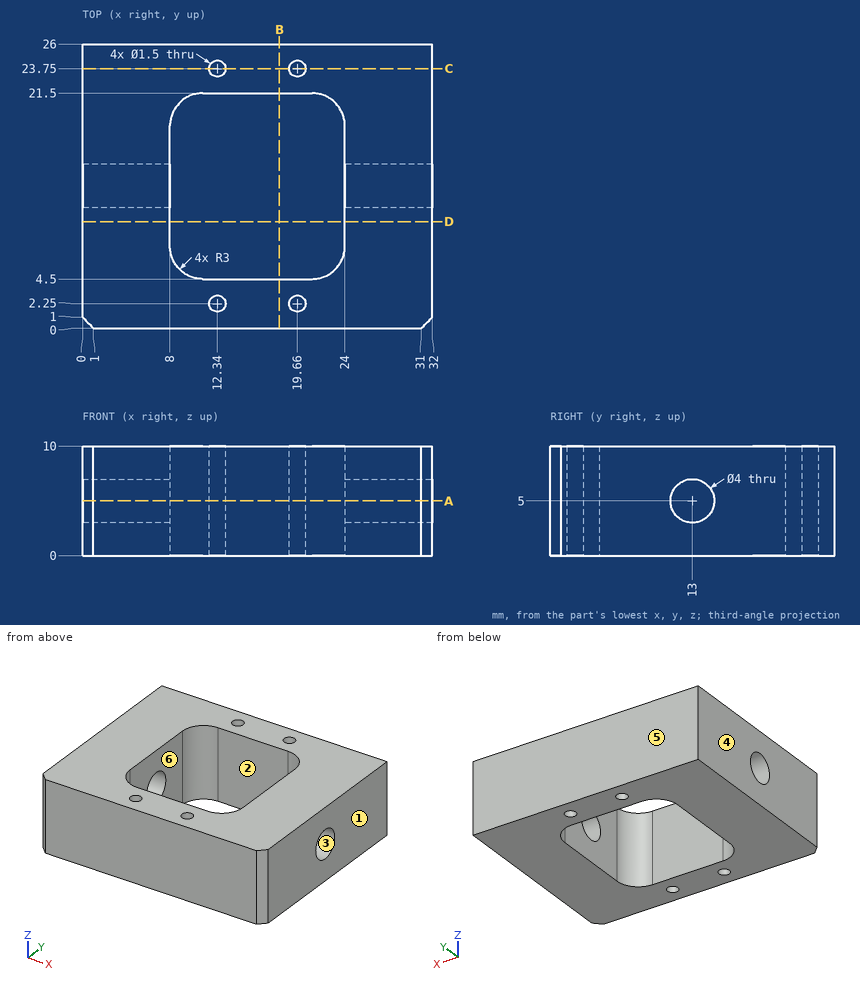
Can you work these out from the drawing? Everything is in mm from the part's minimum corner. A direction names the side the tool comes from. Give positions to 0.01 mm unless a question says otherwise; leave off trailing zeros. Write each loop counter-clockwise with the first axis right and the second up, starting at its lowest first coordinate (ties: lowest second). Pieces come first, ordered by that corner, then holes. Notation, with made-up numbers: M -23,78.5 L 24,78.5 A22 cw 24,87.5 Z; hole C 22,-24.5 d10. An arc over 180 degrees is marked long. Answer in a Markdown table with one row per item. Add a question column.
Item 1: On a 3-axis mill with a long thin cutter (end or side, diameter ignored), from which of +Z, -Z, +X, -X, +Y, -Y can I reach the whole of each face in a straight line? I mean the marked faces 5 and 6. Say none if no direction works.
Item 2: Imagine slicing it at B-B, the plane x = 18. Write out the boundary of the cut face in (y, z).
Item 3: Imagine slicing it at D-D, the plane y = 9.75. Write out the boundary of the cut face in (x, z).
Item 4: Imagine slicing it at A-A, the plane z = 5. Write out the boundary of the cut face in (x, y), plus the area to 3 significant figures.
Item 5: We'd pull the mould along X, two halves only. Please class the marked faces 1, 2, 3 and 4: released by +X, released by -X, zero draft, split by the parting line, or undercut.
Item 6: Please list where these lines run through material, in increasing order: L1, parallel to Y at x = 19.66, z = 4.25; L2, parallel to X at y = 15, z = 6.25; L3, parallel to Y at x = 21, z = 6.5.
Item 7: Imagine slicing it at C-C, the plane y = 23.75. Write out the boundary of the cut face in (x, z), plus the area to 3 significant figures.
Evaluation:
| question | item | result |
|---|---|---|
| 1 | face 5 | +Z, -Z, +X, -X, +Y |
| 1 | face 6 | +Z, -Z |
| 2 | outline | M 0,0 L 4.5,0 L 4.5,10 L 0,10 Z; M 21.5,0 L 26,0 L 26,10 L 21.5,10 Z |
| 3 | outline | M 0,0 L 8,0 L 8,10 L 0,10 Z; M 24,0 L 32,0 L 32,10 L 24,10 Z |
| 4 | outline | M 0,1 L 1,0 L 31,0 L 32,1 L 32,11 L 24,11 L 24,7.5 A3 cw 21,4.5 L 11,4.5 A3 cw 8,7.5 L 8,11 L 0,11 Z; M 0,15 L 8,15 L 8,18.5 A3 cw 11,21.5 L 21,21.5 A3 cw 24,18.5 L 24,15 L 32,15 L 32,26 L 0,26 Z; hole C 12.34,2.25 d1.5; hole C 12.34,23.75 d1.5; hole C 19.66,2.25 d1.5; hole C 19.66,23.75 d1.5 |
| 4 | area | 496 mm² |
| 5 | face 1 | released by +X |
| 5 | face 2 | undercut |
| 5 | face 3 | zero draft |
| 5 | face 4 | released by -X |
| 6 | L1 | y = 0 to 1.5, 3 to 4.5, 21.5 to 23, 24.5 to 26 |
| 6 | L2 | x = 0 to 8, 24 to 32 |
| 6 | L3 | y = 0 to 4.5, 21.5 to 26 |
| 7 | outline | M 0,0 L 11.59,0 L 11.59,10 L 0,10 Z; M 13.09,0 L 18.91,0 L 18.91,10 L 13.09,10 Z; M 20.41,0 L 32,0 L 32,10 L 20.41,10 Z |
| 7 | area | 290 mm² |
